```python
from build123d import *

# Parameters (mm, degrees)
F1_DEPTH = 350
F2_W     = 3
F2_H     = 15
F7_COUNT = 6
F7_ANGLE = 300


with BuildPart() as f1:
    # F0 (on Top) → F1 (new body)
    with BuildSketch(Plane.XY):
        with BuildLine():
            ThreePointArc((5, 257), (-3.535534, 260.535534), (0, 252))
            ThreePointArc((0, 252), (3.535534, 253.464466), (5, 257))
        make_face()
    extrude(amount=F1_DEPTH)


with BuildPart() as f1_1:
    # F5: moved
    add(f1.part.moved(Location((0, 0, -20))))

    # F2 (on Right) → F6 (revolve)
    with BuildSketch(Plane.YZ):
        with Locations((262.5, 7.5)):
            Rectangle(F2_W, F2_H)
    revolve(axis=Axis((0, 0, -57.719678), (0, 0, -1)))

    # F7: F1 ×6 about axis
    f7_axis = Axis((0, 0, -44.895653), (0, 0, -1))


with BuildPart() as f1_2:
    add(f1_1.part)
    for i in range(1, F7_COUNT):
        add(f1_1.part.rotate(f7_axis, i * F7_ANGLE / (F7_COUNT - 1)))


solid = f1_2.part
```
The model under review builds one solid part; all positions refer to its coordinate system, in mm. Round coordinates to 2 decimals unless told otherwise and drop trailing zeros. Order: outer loops, then holes, each group sorted by start corner. A loop starts at its lowest first (then second) coordinate and runs counter-clockwise, first axis right, second up. Notation, with made-up numbers: (8, -38.75) -> (66, -38.75) arc R22 ccw to (66, -21.75) -> close; hole circle Ø2 at (53, -6.75). An arc over 180 degrees is marked (long way). Use a Markdown table: item, result.
Q1. For line 1 (X direction, y = 132, z = 140), list the stretches that pass through material, from the lowest coordinate up.
Values:
| item | result |
|---|---|
| line 1 | x = -226.14 to -219, 219 to 226.14 |
Q2. We need section A-A on y = 0. Write out the cut boundary in (x, z).
Values:
| item | result |
|---|---|
| outline | (-264, 0) -> (-261, 0) -> (-261, 15) -> (-264, 15) -> close; (261, 0) -> (264, 0) -> (264, 15) -> (261, 15) -> close |
Q3. We need section B-B on z = 113. Write out the cut boundary in (x, y).
Values:
| item | result |
|---|---|
| outline | circle Ø10 at (-222.57, -128.5); circle Ø10 at (-222.57, 128.5); circle Ø10 at (0, -257); circle Ø10 at (0, 257); circle Ø10 at (222.57, -128.5); circle Ø10 at (222.57, 128.5) |
Q4. Clearance check with a flat-ended pin moving along its axis: P1, Ø8, axis at y = -120.5, z = 251, coming from the +X side. State where the tip first meets the part, or that it passes through.
Values:
| item | result |
|---|---|
| P1 | stops at x = 225.57 |
Q5. Mouldability with a two-part tool opening along Y and no side actions: class faces 1 (the flat face through (60, 255, 0)), 2 (the cylindrical face through (-101.11, 243.87, 7.6)), 3 (the cylindrical face through (-132.1, 225.1, 7.6)) as +Y half, -Y half, draft (parallel to the pull), parting line (faces both ways), or undercut.
Values:
| item | result |
|---|---|
| face 1 | draft |
| face 2 | parting line |
| face 3 | undercut |
Q6. We need section C-C on x = -79. Write out the cut boundary in (y, z), then the cut area to 3 significant figures.
Values:
| item | result |
|---|---|
| outline | (-251.9, 0) -> (-248.76, 0) -> (-248.76, 15) -> (-251.9, 15) -> close; (248.76, 0) -> (251.9, 0) -> (251.9, 15) -> (248.76, 15) -> close |
| area | 94.4 mm^2 |
